Check sheet for the modelled part. Datum: model origin and axes. Units: mm. Face numbers are marked on the shaded views. A direction names the side the tool comes from. Round coordinates to 2 decimals unless told otherwise and drop trailing zeros. Order: outer loops, then holes, each group sorted by start corner. A loop starts at its lowest first (then second) coordinate and runs counter-clockwise, first axis right, second up. Notation, with made-up numbers: M 62,-15.75 L 86,-15.75 A21 cw 86,5.25 Z; hole C -18,57.5 d8. An arc over 180 degrees is marked long. One line per item, written item: value. Start each with the question number.
(1) Cross-section at C-C, the plane y = 50. Enter the section's corners in (x, z).
(2) Access from +Z, -Z, +X, -X, +Y, -Y to the whole of each face (thin tool, end or side, straight path). Record for the marked faces 1 and 2.
(3) Cross-section at D-D, the plane y = 12. Enter the section's corners in (x, z), and give its area (3 significant figures).
(4) Cross-section at B-B, the plane z = -2.1. Enter the section's corners in (x, y), and give its area (3 significant figures).
(5) Cross-section at A-A, the plane x = 43. Enter the section's corners in (y, z).
(6) Thickness scan on L1, parallel to X at y = 34, z = -0.15; L2, parallel to Y at x = 43, z = 0.8; L3, parallel to Z at x = 20.5, y = 34. Record the ranges inside material, lowest first.
(7) Depth check by flat-ended pin: pin 1 Ø1.8 at (y, z) = (34.5, 0.5) entering from +X; pin 2 Ø1 at (x, y) = (16.5, 15) entering from -Z; pin 3 Ø2 at (x, z) = (34.5, 0.5) entering from -Y. Enter the tip coordinate at first touch or a pass-through.
from build123d import *

# Parameters (mm, degrees)
SKETCH1_R           = 2.7
BOSS_EXTRUDE1_DEPTH = 3
SKETCH2_W           = 30
SKETCH2_H           = 56
SKETCH2_W_2         = 20
SKETCH2_H_2         = 46
BOSS_EXTRUDE2_DEPTH = 3
FILLET1_R           = 4
FILLET3_R           = 1


with BuildPart() as part:
    # Sketch1 → Boss-Extrude1 (new body)
    with BuildSketch(Plane.XY):
        Polygon((0, 0), (0, 56), (50.5, 56), (50.5, 41), (30, 41), (30, 0), align=None)
        with Locations((43, 50)):
            Circle(SKETCH1_R, mode=Mode.SUBTRACT)
    extrude(amount=BOSS_EXTRUDE1_DEPTH)

    # Sketch2 → Boss-Extrude2 (add)
    with BuildSketch(Plane(origin=(0, 0, 0), x_dir=(-1, 0, 0), z_dir=(0, 0, -1))):
        with Locations((-15, 28)):
            Rectangle(SKETCH2_W, SKETCH2_H)
        with Locations((-15, 28)):
            Rectangle(SKETCH2_W_2, SKETCH2_H_2, mode=Mode.SUBTRACT)
    extrude(amount=BOSS_EXTRUDE2_DEPTH)

    # Fillet1
    fillet1_edges = [part.edges().sort_by_distance(p)[0] for p in [
        (50.5, 56, 1.5),
        (50.5, 41, 1.5),
    ]]
    fillet(fillet1_edges, radius=FILLET1_R)

    # Fillet3
    fillet3_edges = [part.edges().sort_by_distance(p)[0] for p in [
        (0, 0, 0),
        (0, 56, 0),
        (30, 0, 0),
        (30, 56, -1.5),
    ]]
    fillet(fillet3_edges, radius=FILLET3_R)


solid = part.part
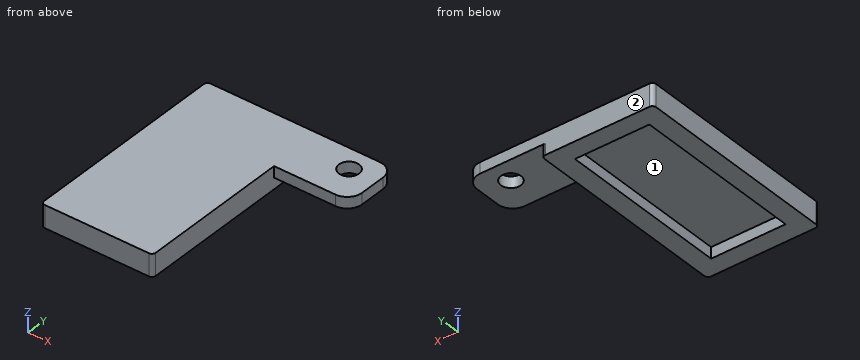
Values found:
1. outline: M 0,-3 L 5,-3 L 5,0 L 25,0 L 25,-3 L 30,-3 L 30,0 L 40.3,0 L 40.3,3 L 0,3 Z; M 45.7,0 L 50.5,0 L 50.5,3 L 45.7,3 Z
2. face 1: -Z
2. face 2: +Z, -Z, +X, -X, +Y
3. outline: M 0,-3 L 5,-3 L 5,0 L 25,0 L 25,-3 L 30,-3 L 30,3 L 0,3 Z
3. area: 120 mm^2
4. outline: M 0,1 A1 ccw 1,0 L 29,0 A1 ccw 30,1 L 30,55 A1 ccw 29,56 L 1,56 A1 ccw 0,55 Z; hole M 5,5 L 25,5 L 25,51 L 5,51 Z
4. area: 759 mm^2
5. outline: M 41,0 L 47.3,0 L 47.3,3 L 41,3 Z; M 52.7,0 L 56,0 L 56,3 L 52.7,3 Z
6. L1: 0 to 5, 25 to 30
6. L2: 41 to 47.3, 52.7 to 56
6. L3: 0 to 3
7. pin 1: x = 30
7. pin 2: z = 0
7. pin 3: y = 41
